Autodesk Fusion 360 part; units mm, degrees
sketch "Sketch1" plane through (0, 0, 0) normal (0, 0, 1) x (1, 0, 0)
  line L0 (0, 0) -> (-38.1, 0)
  line L1 (-38.1, 0) -> (-38.1, 38.1)
  line L2 (-38.1, 38.1) -> (0, 38.1)
  line L3 (0, 38.1) -> (0, 0)
  dimension "d1" = 38.1
  dimension "d2" = 38.1
extrude "Extrude1" add sketch "Sketch1" along normal blind 25.4
chamfer "Chamfer1" distance 15.24 angle 45 2 edges at (-19.05, 0, 25.4) (-19.05, 38.1, 25.4)
sketch "Sketch2" plane through (0, 0, 25.4) normal (0, 0, 1) x (-1, 0, 0)
  line L0 (0, -22.86) -> (38.1, -22.86)
  line L1 (38.1, -22.86) -> (38.1, -15.24)
  line L2 (38.1, -15.24) -> (0, -15.24)
  line L3 (0, -15.24) -> (0, -22.86)
  line L4 (38.1, -19.05) -> (0, -19.05)
  line L5 (0, -19.05) -> (0, -20.6375)
  line L6 (0, -20.6375) -> (38.1, -20.6375)
  line L7 (38.1, -20.6375) -> (38.1, -19.05)
  line L8 (38.1, -19.05) -> (0, -19.05)
  line L9 (0, -19.05) -> (0, -17.4625)
  line L10 (0, -17.4625) -> (38.1, -17.4625)
  line L11 (38.1, -17.4625) -> (38.1, -19.05)
  dimension "d6" = 1.5875
  dimension "d7" = 1.5875
extrude "Extrude2" cut sketch "Sketch2" against normal blind 19.05 contours L1 L3 L4 L5 L6 L7 L8 | L1 L3 L4 L8 L9 L10 L11
sketch "Sketch3" plane through (0, 0, 0) normal (0, 0, -1) x (1, 0, 0)
  line L0 (-38.1, -38.1) -> (0, -38.1)
  line L1 (0, -38.1) -> (0, 0)
  line L2 (0, 0) -> (-38.1, 0)
  line L3 (-38.1, 0) -> (-38.1, -38.1)
  circle A0 centre (-19.05, -19.05) radius 15.875
  dimension "d10" = 31.75
extrude "Extrude3" cut sketch "Sketch3" against normal blind 3.175 contours A0
Geometry: final body of the model. Coordinates: model frame, mm. A direction names the side the tool comes from. Coordinates: 2 decimals unless noted, no trailing zeros. Write each loop counter-clockwise with the first axis right and the second up, starting at its lowest first coordinate (ties: lowest second). Pieces come first, ordered by that corner, then holes. Notation, with made-up numbers: M -26.5,15.5 L -21.5,15.5 A20 cw -21.5,53.5 Z; hole C 31.25,42.5 d3. An arc over 180 degrees is marked long. Use CSV: the item, a comma, the result in double quotes. Start each with the question number.
1. Ray query, probe 1 along Y at (x, z) = (-19.05, 2.45) (3 decimals); probe 2 along X at (y, z) = (19.05, 1.3) (3 decimals); probe 3 along Y at (x, z) = (-25, 9.75). Return the intervals inside material, ascending.
2. Cut plane A-A on z = 15.5. Return the cut outline in (x, y), plus the area to 3 significant figures.
3. Mould query, pull axis Y, two halves, no side actions, for faces 4 (the face through (-19, 16, 25.4)), 5 (the face through (-19, 19, 3.175)), 6 (the face through (-19, 19, 6.35)), 7 (the face through (-19, 0, 5)). Classes: pulls with the +Y half, pulls with the -Y half, needs draft (parallel to the pull), parting line crosses it, or undercut.
4. Reachability of faces 1 (the face through (-19, 20.638, 16)), 2 (the face through (-22.491, 34.547, 1.565)), 3 (the face through (-38.1, 23, 10)) from +Z, -Z, +X, -X, +Y, -Y: full face, straight path, thin tool, end or side. Return the list, or none.
5. Cut plane B-B on z = 1.5. Return the cut outline in (x, y) (3 decimals), plus the area to 3 significant figures.
6. Cut plane C-C on y = 19.05. Return the cut outline in (x, z) (3 decimals).
7. First-contact query: P1, Ø1.5, axis at x = -8.5, z = 15.5, coming from the +Y side; P2, Ø1, axis at x = -14, y = 28.5, coming from the +Z side; P3, Ø9.5, axis at x = -16.5, z = 20.5, coming from the -Y side. Flat tips, straight axial feed; report the tip coordinate or a pass-through.
Entries:
1,probe 1,"0 to 3.175, 34.925 to 38.1"
1,probe 2,"-38.1 to -34.925, -3.175 to 0"
1,probe 3,"0 to 17.46, 20.64 to 38.1"
2,outline,"M -38.1,5.34 L 0,5.34 L 0,17.46 L -38.1,17.46 Z; M -38.1,20.64 L 0,20.64 L 0,32.76 L -38.1,32.76 Z"
2,area,"924 mm²"
3,face 4,"needs draft"
3,face 5,"undercut"
3,face 6,"undercut"
3,face 7,"pulls with the -Y half"
4,face 1,"+Z, +X, -X"
4,face 2,"-Z"
4,face 3,"+Z, -Z, -X, +Y, -Y"
5,outline,"M -38.1,0 L 0,0 L 0,38.1 L -38.1,38.1 Z; hole C -19.05,19.05 d31.75"
5,area,"660 mm²"
6,outline,"M -38.1,0 L -34.925,0 L -34.925,3.175 L -3.175,3.175 L -3.175,0 L 0,0 L 0,6.35 L -38.1,6.35 Z"
7,P1,"y = 33.51"
7,P2,"z = 20.26"
7,P3,"y = 5.59"
